Model file for the job. Use its own axes, mm. A direction names the side the tool comes from. Round coordinates to 2 decimals unless told otherwise and drop trailing zeros. Write each loop counter-clockwise with the first axis right and the second up, starting at its lowest first coordinate (ties: lowest second). Pieces come first, ordered by that corner, then holes.
```python
from build123d import *

# Parameters (mm, degrees)
BOSS_EXTRUDE1_DEPTH  = 112
SKETCH2_R            = 19.05
BOSS_EXTRUDE2_DEPTH  = 1.6
SKETCH3_R            = 4
BOSS_EXTRUDE3_DEPTH  = 19.4
SKETCH4_W            = 7.896046337
SKETCH4_H            = 7.324948646
CUT_EXTRUDE1_DEPTH   = 19.4
CUT_EXTRUDE2_DEPTH   = 107.2
MIRROR2_COPY_1_DEPTH = 107.2
FILLET1_R            = 3
SKETCH6_R            = 2.5
CUT_EXTRUDE3_DEPTH   = 107.2


with BuildPart() as part:
    # Sketch1 → Boss-Extrude1 (new body)
    with BuildSketch(Plane(origin=(0, 0, 0), x_dir=(1, 0, 0), z_dir=(0, 1, 0))):
        with BuildLine():
            Line((-24.5, -28.5), (24.5, -28.5))
            ThreePointArc((24.5, -28.5), (27.328427125, -27.328427125), (28.5, -24.5))
            Line((28.5, -24.5), (28.5, 24.5))
            ThreePointArc((28.5, 24.5), (27.328427125, 27.328427125), (24.5, 28.5))
            Line((24.5, 28.5), (-24.5, 28.5))
            ThreePointArc((-24.5, 28.5), (-27.328427125, 27.328427125), (-28.5, 24.5))
            Line((-28.5, 24.5), (-28.5, -24.5))
            ThreePointArc((-28.5, -24.5), (-27.328427125, -27.328427125), (-24.5, -28.5))
        make_face()
    extrude(amount=BOSS_EXTRUDE1_DEPTH)

    # Sketch2 → Boss-Extrude2 (add)
    with BuildSketch(Plane(origin=(0, 112, 0), x_dir=(1, 0, 0), z_dir=(0, 1, 0))):
        Circle(SKETCH2_R)
    extrude(amount=BOSS_EXTRUDE2_DEPTH)

    # Sketch3 → Boss-Extrude3 (add)
    with BuildSketch(Plane(origin=(0, 113.6, 0), x_dir=(1, 0, 0), z_dir=(0, 1, 0))):
        Circle(SKETCH3_R)
    extrude(amount=BOSS_EXTRUDE3_DEPTH)

    # Sketch4 → Cut-Extrude1 (cut)
    with BuildSketch(Plane(origin=(0, 133, 0), x_dir=(1, 0, 0), z_dir=(0, 1, 0))):
        with Locations((6.304367274, 0.076945889)):
            Rectangle(SKETCH4_W, SKETCH4_H)
    extrude(amount=-CUT_EXTRUDE1_DEPTH, mode=Mode.SUBTRACT)

    # Sketch5 → Cut-Extrude2 (cut)
    with BuildSketch(Plane.XZ):
        with BuildLine():
            Line((-28.5, 24.5), (-28.5, 18.683107864))
            Line((-28.5, 18.683107864), (-18.683107864, 18.683107864))
            Line((-18.683107864, 18.683107864), (-18.683107864, 28.5))
            Line((-18.683107864, 28.5), (-24.5, 28.5))
            ThreePointArc((-24.5, 28.5), (-27.328427125, 27.328427125), (-28.5, 24.5))
        make_face()
    cut_extrude2 = extrude(amount=-CUT_EXTRUDE2_DEPTH, mode=Mode.SUBTRACT)

    # Mirror1: Cut-Extrude2 across plane
    add(cut_extrude2.mirror(Plane(origin=(0, 0, 0), x_dir=(0, 0, 1), z_dir=(1, 0, 0))), mode=Mode.SUBTRACT)

    # Mirror2: Cut-Extrude2 across plane
    add(cut_extrude2.mirror(Plane.XY), mode=Mode.SUBTRACT)

    # Mirror2 copy 1 sketch → Mirror2 copy 1 (cut)
    with BuildSketch(Plane(origin=(0, 0, 0), x_dir=(-1, 0, 0), z_dir=(0, -1, 0))):
        with BuildLine():
            Line((-28.5, 24.5), (-28.5, 18.683107864))
            Line((-28.5, 18.683107864), (-18.683107864, 18.683107864))
            Line((-18.683107864, 18.683107864), (-18.683107864, 28.5))
            Line((-18.683107864, 28.5), (-24.5, 28.5))
            ThreePointArc((-24.5, 28.5), (-27.328427125, 27.328427125), (-28.5, 24.5))
        make_face()
    extrude(amount=-MIRROR2_COPY_1_DEPTH, mode=Mode.SUBTRACT)

    # Fillet1
    fillet1_edges = [part.edges().sort_by_distance(p)[0] for p in [
        (-18.683107864, 53.6, -18.683107864),
        (-18.683107864, 53.6, -28.5),
        (-28.5, 53.6, -18.683107864),
        (-18.683107864, 53.6, 28.5),
        (-18.683107864, 53.6, 18.683107864),
        (-28.5, 53.6, 18.683107864),
        (18.683107864, 53.6, 18.683107864),
        (18.683107864, 53.6, 28.5),
        (28.5, 53.6, 18.683107864),
        (18.683107864, 53.6, -28.5),
        (18.683107864, 53.6, -18.683107864),
        (28.5, 53.6, -18.683107864),
    ]]
    fillet(fillet1_edges, radius=FILLET1_R)

    # Sketch6 → Cut-Extrude3 (cut)
    with BuildSketch(Plane(origin=(0, 112, 0), x_dir=(1, 0, 0), z_dir=(0, 1, 0))):
        with Locations((23.5, 23.5)):
            Circle(SKETCH6_R)
        with Locations((23.564387561, -23.499955896)):
            Circle(SKETCH6_R)
        with Locations((-23.5, 23.5)):
            Circle(SKETCH6_R)
        with Locations((-23.435612439, -23.5)):
            Circle(SKETCH6_R)
    extrude(amount=-CUT_EXTRUDE3_DEPTH, mode=Mode.SUBTRACT)


solid = part.part
```
1) Cut at D-D on x = 10. List the corners of the cut face in (y, z), and give its area (3 significant figures).
2) Cut at B-B on z = 0. List the corners of the cut face in (x, y).
3) Wall check: probe 1 along X at (y, z) = (108.7, -23.5); probe 2 along Z at (x, y) = (23, 110). Give the ranges that are in metal, low to high.
4) Which spindle directions (+Z, -Z, +X, -X, +Y, -Y) get a long thin tool onto all of the face, cutting with end or side? Do faces 5 (the face through (-15.12, 112.79, 11.59)), 6 (the face through (-18.683, 53, -24)), 7 (the face through (24, 53, -18.683)). Say none if no direction does.
5) Flat gauge pins, fed straight in: pin 1 Ø1.9 at (y, z) = (54.5, -24) entering from -X; pin 2 Ø5 at (y, z) = (120, -1) entering from +X; pin 3 Ø6.5 at (x, z) = (-23.5, -23.5) entering from -Y; pin 4 Ø10 at (y, z) = (118.5, -20.5) entering from +X. Where does each tip first touch, or does it go through?
6) Pull direction X, two halves, no side cores. Call faces 1 (the face through (-22.092, 109.634, 21.392)), 2 (the face through (-17.781, 54.35, 27.645)), 3 (the face through (-24, 53, 18.683)), 4 (the face through (17.781, 54.35, 27.645)): released by +X, released by -X, zero draft, split by the parting line, or undercut.
7) Cut at C-C on y = 16. List the corners of the cut face in (x, z).
8) Cut at A-A on x = 0. List the corners of the cut face in (y, z).
Result sheet:
1. outline: (0, -28.5) - (112, -28.5) - (112, -16.21) - (113.6, -16.21) - (113.6, 16.21) - (112, 16.21) - (112, 28.5) - (0, 28.5) - close
1. area: 6,440 mm2
2. outline: (-28.5, 0) - (28.5, 0) - (28.5, 112) - (19.05, 112) - (19.05, 113.6) - (2.36, 113.6) - (2.36, 133) - (-4, 133) - (-4, 113.6) - (-19.05, 113.6) - (-19.05, 112) - (-28.5, 112) - close
3. probe 1: x = -28.5 to -26, -21 to 21, 26 to 28.5
3. probe 2: z = -28.5 to -25.95, -21.05 to 21.06, 25.94 to 28.5
4. face 5: +Y
4. face 6: -Z, -X, -Y
4. face 7: -Z, +X, -Y
5. pin 1: stops at x = -18.68
5. pin 2: stops at x = 2.36
5. pin 3: stops at y = 107.2
5. pin 4: passes through
6. face 1: undercut
6. face 2: released by -X
6. face 3: zero draft
6. face 4: released by +X
7. outline: (-28.5, -15.68) arc R3 ccw to (-25.5, -18.68) - (-21.68, -18.68) arc R3 cw to (-18.68, -21.68) - (-18.68, -25.5) arc R3 ccw to (-15.68, -28.5) - (15.68, -28.5) arc R3 ccw to (18.68, -25.5) - (18.68, -21.68) arc R3 cw to (21.68, -18.68) - (25.5, -18.68) arc R3 ccw to (28.5, -15.68) - (28.5, 15.68) arc R3 ccw to (25.5, 18.68) - (21.68, 18.68) arc R3 cw to (18.68, 21.68) - (18.68, 25.5) arc R3 ccw to (15.68, 28.5) - (-15.68, 28.5) arc R3 ccw to (-18.68, 25.5) - (-18.68, 21.68) arc R3 cw to (-21.68, 18.68) - (-25.5, 18.68) arc R3 ccw to (-28.5, 15.68) - close
8. outline: (0, -28.5) - (112, -28.5) - (112, -19.05) - (113.6, -19.05) - (113.6, -4) - (133, -4) - (133, 4) - (113.6, 4) - (113.6, 19.05) - (112, 19.05) - (112, 28.5) - (0, 28.5) - close
